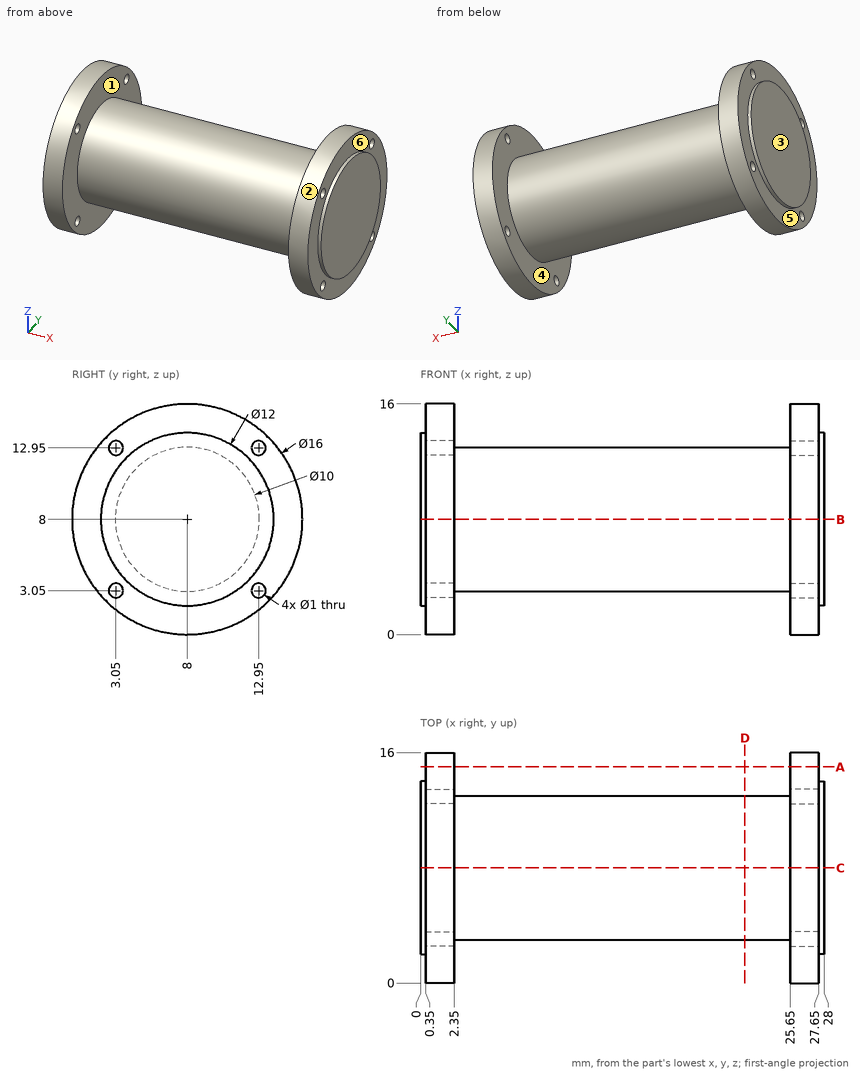
Verification items for this drawing (mm, ordinates from the low corner). A direction names the side the tool comes from. Round coordinates to 2 decimals unless told otherwise and drop trailing zeros. Order: outer loops, then holes, each group sorted by start corner. A loop starts at its lowest first (then second) coordinate and runs counter-clockwise, first axis right, second up. Notation, with made-up numbers: (45.5, 11.25) - (89.5, 11.25) arc R36 ccw to (89.5, 48.25) - close; hole circle Ø5 at (-17, 66). An arc over 180 degrees is marked (long way). Use CSV: the item, a comma, the result in double quotes. Start each with the question number.
1) Access from +Z, -Z, +X, -X, +Y, -Y to the whole of each face (thin tool, end or side, straight path). Record for the marked faces 4, 5 and 6.
2) Section check A-A, the plane y = 15. Record the cut outline in (x, z), plus the area to 3 significant figures.
3) Thickness scan on L1, parallel to X at y = 5.5, z = 3.5; L2, parallel to X at y = 2, z = 6.5; L3, parallel to Z at x = 11.25, y = 7.5 (1 decimal). Record the ranges inside material, lowest first.
4) Section check B-B, the plane z = 8. Record the cut outline in (x, y), plus the area to 3 significant figures.
5) Section check D-D, the plane x = 22.5. Record the cut outline in (y, z).
6) Go/stop test with flat-tipped pins: P1, Ø8, axis at x = 12, z = 8.5, coming from the -Y side; P2, Ø1.5, axis at x = 8.5, z = 9.5, coming from the +Y side; P3, Ø3, axis at x = 8, z = 11, coming from the -Y side. Record where each tip stops, or that it passes through.
7) Mould release check, pull along X, two halves, no side actions. Record for the marked faces 1, 2 and 3: +X half, -X half, draft (parallel to the pull), parting line (faces both ways), or undercut.
Answers:
1,face 4,"none"
1,face 5,"-X"
1,face 6,"+X"
2,outline,"(0.35, 4.13) - (2.35, 4.13) - (2.35, 11.87) - (0.35, 11.87) - close; (25.65, 4.13) - (27.65, 4.13) - (27.65, 11.87) - (25.65, 11.87) - close"
2,area,"31.0 mm²"
3,L1,"x = 0 to 2.35, 25.65 to 28"
3,L2,"x = 0.35 to 2.35, 25.65 to 27.65"
3,L3,"z = 3 to 13"
4,outline,"(0, 2) - (0.35, 2) - (0.35, 0) - (2.35, 0) - (2.35, 3) - (25.65, 3) - (25.65, 0) - (27.65, 0) - (27.65, 2) - (28, 2) - (28, 14) - (27.65, 14) - (27.65, 16) - (25.65, 16) - (25.65, 13) - (2.35, 13) - (2.35, 16) - (0.35, 16) - (0.35, 14) - (0, 14) - close"
4,area,"305 mm²"
5,outline,"circle Ø10 at (8, 8)"
6,P1,"stops at y = 3"
6,P2,"stops at y = 12.94"
6,P3,"stops at y = 3.23"
7,face 1,"undercut"
7,face 2,"draft"
7,face 3,"-X half"
